Check sheet for the modelled part. Datum: model origin and axes. Units: mm. Give positions to 0.01 mm unless a question says otherwise; leave off trailing zeros. Order: outer loops, then holes, each group sorted by start corner. A loop starts at its lowest first (then second) coordinate and runs counter-clockwise, first axis right, second up. Notation, with made-up numbers: M 10,4.5 L 17,4.5 A29 cw 17,30.5 Z; hole C -21.5,3.5 d7. An arc over 180 degrees is marked long. Return JSON: item names as keys, results as strings. Group by question number.
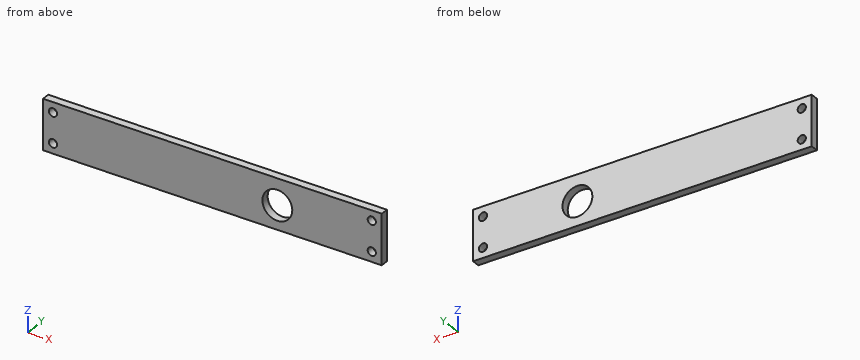
from build123d import *

# Parameters (mm, degrees)
SKETCH1_W           = 136
SKETCH1_H           = 20
SKETCH1_R           = 1.65
SKETCH1_R_2         = 6
BOSS_EXTRUDE1_DEPTH = 3.175


with BuildPart() as part:
    # Sketch1 → Boss-Extrude1 (new body)
    with BuildSketch(Plane(origin=(0, 0, 0), x_dir=(1, 0, 0), z_dir=(0, 1, 0))):
        with Locations((68, -10)):
            Rectangle(SKETCH1_W, SKETCH1_H)
        with Locations(Location((4, -4, 0), (0, 0, 270))):
            Circle(SKETCH1_R, mode=Mode.SUBTRACT)
        with Locations(Location((132, -4, 0), (0, 0, 270))):
            Circle(SKETCH1_R, mode=Mode.SUBTRACT)
        with Locations(Location((94.08554011, -9.52416591, 0), (0, 0, 270))):
            Circle(SKETCH1_R_2, mode=Mode.SUBTRACT)
        with Locations(Location((4, -16, 0), (0, 0, 270))):
            Circle(SKETCH1_R, mode=Mode.SUBTRACT)
        with Locations(Location((132, -16, 0), (0, 0, 270))):
            Circle(SKETCH1_R, mode=Mode.SUBTRACT)
    extrude(amount=BOSS_EXTRUDE1_DEPTH)


solid = part.part
1) Sectioned sample at A-A on x = 132. Record the boundary of the cut face in (y, z) (3 decimals), then the cut area to 3 significant figures.
2) Sectioned sample at C-C on y = 1.75. Record the boundary of the cut face in (x, z).
3) Sectioned sample at B-B on z = 8. Record the boundary of the cut face in (x, y) (3 decimals).
4) Material ranges on line 1 along X through (y, z) = (1.5, 16); line 2 along X through (y, z) = (1.5, 4); line 3 along X through (y, z) = (0.8, 5.25), recorded low to high.
Reply:
{
 "1": {"outline": "M 0,0 L 3.175,0 L 3.175,2.35 L 0,2.35 Z; M 0,5.65 L 3.175,5.65 L 3.175,14.35 L 0,14.35 Z; M 0,17.65 L 3.175,17.65 L 3.175,20 L 0,20 Z", "area": "42.5 mm^2"},
 "2": {"outline": "M 0,0 L 136,0 L 136,20 L 0,20 Z; hole C 4,4 d3.3; hole C 4,16 d3.3; hole C 94.09,9.52 d12; hole C 132,4 d3.3; hole C 132,16 d3.3"},
 "3": {"outline": "M 0,0 L 88.282,0 L 88.282,3.175 L 0,3.175 Z; M 99.889,0 L 136,0 L 136,3.175 L 99.889,3.175 Z"},
 "4": {"line 1": "0 to 2.35, 5.65 to 130.35, 133.65 to 136", "line 2": "0 to 2.35, 5.65 to 91.74, 96.43 to 130.35, 133.65 to 136", "line 3": "0 to 2.92, 5.08 to 89.87, 98.3 to 130.92, 133.08 to 136"}
}
